For this review, take the finished solid that the model builds, in its own axes (mm). A direction names the side the tool comes from. Round coordinates to 2 decimals unless told otherwise and drop trailing zeros. Order: outer loops, then holes, each group sorted by start corner. A loop starts at its lowest first (then second) coordinate and runs counter-clockwise, first axis right, second up. Notation, with made-up numbers: (63.5, -33) -> (76.5, -33) arc R28 cw to (76.5, -11) -> close; hole circle Ø8 at (74, -34). An arc over 180 degrees is marked (long way). Use a Markdown table: item, result. Add a question column.
1) Consider section B-B (x = -3). State the section outline as (y, z) points, plus the area to 3 significant figures.
2) Consider section D-D (y = -7.5). State the section outline as (x, z) points, plus the area to 4 significant figures.
3) Consider section A-A (z = 7.5). State the section outline as (x, y) points.
4) Consider section C-C (y = -12.5). State the section outline as (x, z) points.
5) Machinability: for faces 4 (the face through (2, -17, 7)), 5 (the face through (-4.906, -12, -6)), 6 (the face through (2, -4, 3)), which of the approach directions +Z, -Z, +X, -X, +Y, -Y give a long, thin tool a straight path to every point of the face, cutting with its end or side? Answer none if there is none.
6) Clearance check with flat-ended pins moving along their axes: P1, Ø1.5, axis at x = 10.5, y = -20.5, coming from the +Z side; P2, Ø6.5, axis at y = -12.5, z = 7.5, coming from the +X side; P3, Ø4, axis at x = 1.5, z = 6.5, coming from the -Y side. State where each tip first meets the part, or that it passes through.
7) Wall thickness on line 1 along Z through (x, y) = (-3.5, -12.5); line 2 along X through (y, z) = (-21, -6.75); line 3 along Z through (x, y) = (5.25, -12.5): over which ranges is each line inside the solid? List them lowest first. Write a range as [from, to].
8) Draft analysis for pull direction X (two halves, no side actions). For faces 1 (the face through (12.594, -12, -5)), 2 (the face through (-0.906, -12, -14)), 3 (the face through (2, -8, 7)), state which applies: pulls with the +X half, pulls with the -X half, needs draft (parallel to the pull), parting line crosses it, or undercut.
```python
from build123d import *

# Parameters (mm, degrees)
F0_W     = 4
F0_H     = 3
F0_W_2   = 3
F0_H_2   = 15
F1_DEPTH = 25
F2_W     = 20.5
F2_H     = 9
F3_DEPTH = 9
F4_R     = 3.5
F5_DEPTH = 20.5


with BuildPart() as f1:
    # F0 (on Front) → F1 (new body)
    with BuildSketch(Plane.XZ):
        Polygon((-7.90625, 3), (-7.90625, 0), (-4.90625, 0), (9.59375, 0), (12.59375, 0), (12.59375, 3), align=None)
        Polygon((-4.90625, 0), (-7.90625, 0), (-7.90625, -15), (-4.90625, -15), (-4.90625, -12), align=None)
        with Locations((-2.90625, -13.5)):
            Rectangle(F0_W, F0_H)
        with Locations((11.09375, -7.5)):
            Rectangle(F0_W_2, F0_H_2)
    extrude(amount=F1_DEPTH)

    # F2 (on face) → F3 (join)
    with BuildSketch(Plane.XY.offset(3)):
        with Locations((2.34375, -12.5)):
            Rectangle(F2_W, F2_H)
    extrude(amount=F3_DEPTH)

    # F4 (on face) → F5 (cut)
    with BuildSketch(Plane(origin=(-7.90625, 0, 0), x_dir=(0, -1, 0), z_dir=(-1, 0, 0))):
        with Locations((12.5, 7.5)):
            Circle(F4_R)
    extrude(amount=-F5_DEPTH, mode=Mode.SUBTRACT)


solid = f1.part
```
Results list:
| question | item | result |
|---|---|---|
| 1 | outline | (-25, -15) -> (0, -15) -> (0, -12) -> (-25, -12) -> close; (-25, 0) -> (0, 0) -> (0, 3) -> (-8, 3) -> (-8, 12) -> (-17, 12) -> (-17, 3) -> (-25, 3) -> close; hole circle Ø7 at (-12.5, 7.5) |
| 1 | area | 193 mm2 |
| 2 | outline | (-7.91, -15) -> (-0.91, -15) -> (-0.91, -12) -> (-4.91, -12) -> (-4.91, 0) -> (9.59, 0) -> (9.59, -15) -> (12.59, -15) -> (12.59, 3) -> (-7.91, 3) -> close |
| 2 | area | 163.5 mm2 |
| 3 | outline | (-7.91, -17) -> (12.59, -17) -> (12.59, -16) -> (-7.91, -16) -> close; (-7.91, -9) -> (12.59, -9) -> (12.59, -8) -> (-7.91, -8) -> close |
| 4 | outline | (-7.91, -15) -> (-0.91, -15) -> (-0.91, -12) -> (-4.91, -12) -> (-4.91, 0) -> (9.59, 0) -> (9.59, -15) -> (12.59, -15) -> (12.59, 4) -> (-7.91, 4) -> close; (-7.91, 11) -> (12.59, 11) -> (12.59, 12) -> (-7.91, 12) -> close |
| 5 | face 4 | +Z, +X, -X, -Y |
| 5 | face 5 | +Y, -Y |
| 5 | face 6 | +Z, +X, -X, +Y |
| 6 | P1 | z = 3 |
| 6 | P2 | through |
| 6 | P3 | y = -17 |
| 7 | line 1 | [-15, -12], [0, 4], [11, 12] |
| 7 | line 2 | [-7.91, -4.91], [9.59, 12.59] |
| 7 | line 3 | [0, 4], [11, 12] |
| 8 | face 1 | pulls with the +X half |
| 8 | face 2 | undercut |
| 8 | face 3 | needs draft |
